The model under review builds one solid part; all positions refer to its coordinate system, in mm. Round coordinates to 2 decimals unless told otherwise and drop trailing zeros. Loops run counter-clockwise (first coordinate to the right, second up) from the corner with the lowest first, then second, coordinate; pieces in that order, holes last. Notation, with made-up numbers: (-15, -13.75) -> (32, -13.75) arc R33 ccw to (32, 19.25) -> close; hole circle Ø8 at (15, 63.25). An arc over 180 degrees is marked (long way). Use a Markdown table: item, result. Add a question column.
1) Wall thickness on probe 1 along X at (y, z) = (1.75, 9) (3 decimals); probe 2 along Z at (x, y) = (8, 1.5); probe 3 along X at (y, z) = (6.25, 7) (3 decimals): over which ranges is each line inside the solid? List them lowest first.
2) Consider section B-B on x = 27. Give the boundary of the cut face in (y, z), plus the area to 3 significant figures.
3) Consider section A-A on z = 30.5. Give the boundary of the cut face in (x, y) (3 decimals), plus the area to 3 significant figures.
4) Consider section C-C on y = 3.25. State how many separate pieces and enclosed holes the cut face has, plus the area to 3 significant figures.
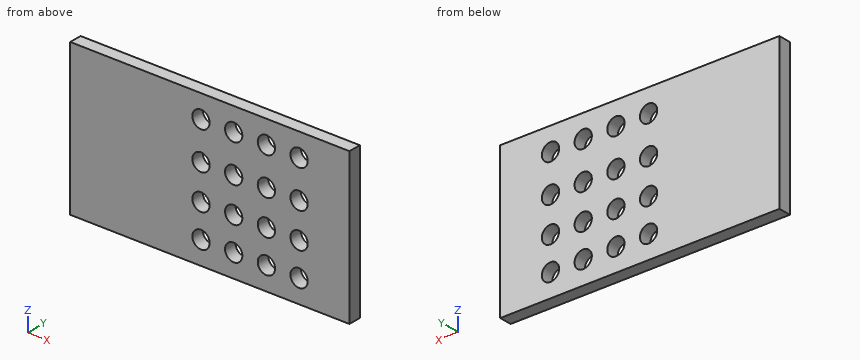
from build123d import *

# Parameters (mm, degrees)
SKETCH1_W           = 140.97
SKETCH1_H           = 76.2
SKETCH1_R           = 4.365625
BOSS_EXTRUDE1_DEPTH = 6.35


with BuildPart() as part:
    # Sketch1 → Boss-Extrude1 (new body)
    with BuildSketch(Plane(origin=(0, 0, 0), x_dir=(1, 0, 0), z_dir=(0, 1, 0))):
        with Locations((-20.32, -1.14427)):
            Rectangle(SKETCH1_W, SKETCH1_H)
        with Locations(Location((-24.765, 25.36698, 0), (0, 0, 270))):
            Circle(SKETCH1_R, mode=Mode.SUBTRACT)
        with Locations(Location((-8.255, 25.36698, 0), (0, 0, 270))):
            Circle(SKETCH1_R, mode=Mode.SUBTRACT)
        with Locations(Location((8.255, 25.36698, 0), (0, 0, 270))):
            Circle(SKETCH1_R, mode=Mode.SUBTRACT)
        with Locations(Location((24.765, 25.36698, 0), (0, 0, 270))):
            Circle(SKETCH1_R, mode=Mode.SUBTRACT)
        with Locations(Location((24.765, 8.78078, 0), (0, 0, 270))):
            Circle(SKETCH1_R, mode=Mode.SUBTRACT)
        with Locations(Location((8.255, 8.78078, 0), (0, 0, 270))):
            Circle(SKETCH1_R, mode=Mode.SUBTRACT)
        with Locations(Location((-8.255, 8.78078, 0), (0, 0, 270))):
            Circle(SKETCH1_R, mode=Mode.SUBTRACT)
        with Locations(Location((-24.765, 8.78078, 0), (0, 0, 270))):
            Circle(SKETCH1_R, mode=Mode.SUBTRACT)
        with Locations(Location((-24.765, -8.78078, 0), (0, 0, 270))):
            Circle(SKETCH1_R, mode=Mode.SUBTRACT)
        with Locations(Location((-8.255, -8.78078, 0), (0, 0, 270))):
            Circle(SKETCH1_R, mode=Mode.SUBTRACT)
        with Locations(Location((8.255, -8.78078, 0), (0, 0, 270))):
            Circle(SKETCH1_R, mode=Mode.SUBTRACT)
        with Locations(Location((24.765, -8.78078, 0), (0, 0, 270))):
            Circle(SKETCH1_R, mode=Mode.SUBTRACT)
        with Locations(Location((24.765, -27.65552, 0), (0, 0, 270))):
            Circle(SKETCH1_R, mode=Mode.SUBTRACT)
        with Locations(Location((8.255, -27.65552, 0), (0, 0, 270))):
            Circle(SKETCH1_R, mode=Mode.SUBTRACT)
        with Locations(Location((-8.255, -27.65552, 0), (0, 0, 270))):
            Circle(SKETCH1_R, mode=Mode.SUBTRACT)
        with Locations(Location((-24.765, -27.65552, 0), (0, 0, 270))):
            Circle(SKETCH1_R, mode=Mode.SUBTRACT)
    extrude(amount=BOSS_EXTRUDE1_DEPTH)


solid = part.part
Result set:
| question | item | result |
|---|---|---|
| 1 | probe 1 | -90.805 to -29.125, -20.405 to -12.615, -3.895 to 3.895, 12.615 to 20.405, 29.125 to 50.165 |
| 1 | probe 2 | -36.96 to -29.73, -21.01 to -13.14, -4.42 to 4.42, 13.14 to 23.3, 32.01 to 39.24 |
| 1 | probe 3 | -90.805 to -28.751, -20.779 to -12.241, -4.269 to 4.269, 12.241 to 20.779, 28.751 to 50.165 |
| 2 | outline | (0, -36.96) -> (6.35, -36.96) -> (6.35, -29.12) -> (0, -29.12) -> close; (0, -21.62) -> (6.35, -21.62) -> (6.35, -12.53) -> (0, -12.53) -> close; (0, -5.03) -> (6.35, -5.03) -> (6.35, 5.03) -> (0, 5.03) -> close; (0, 12.53) -> (6.35, 12.53) -> (6.35, 23.91) -> (0, 23.91) -> close; (0, 31.41) -> (6.35, 31.41) -> (6.35, 39.24) -> (0, 39.24) -> close |
| 2 | area | 293 mm2 |
| 3 | outline | (-90.805, 0) -> (-28.077, 0) -> (-28.077, 6.35) -> (-90.805, 6.35) -> close; (-21.453, 0) -> (-11.567, 0) -> (-11.567, 6.35) -> (-21.453, 6.35) -> close; (-4.943, 0) -> (4.943, 0) -> (4.943, 6.35) -> (-4.943, 6.35) -> close; (11.567, 0) -> (21.453, 0) -> (21.453, 6.35) -> (11.567, 6.35) -> close; (28.077, 0) -> (50.165, 0) -> (50.165, 6.35) -> (28.077, 6.35) -> close |
| 3 | area | 727 mm2 |
| 4 | separate pieces | 1 |
| 4 | enclosed holes | 16 |
| 4 | area | 9,780 mm2 |
